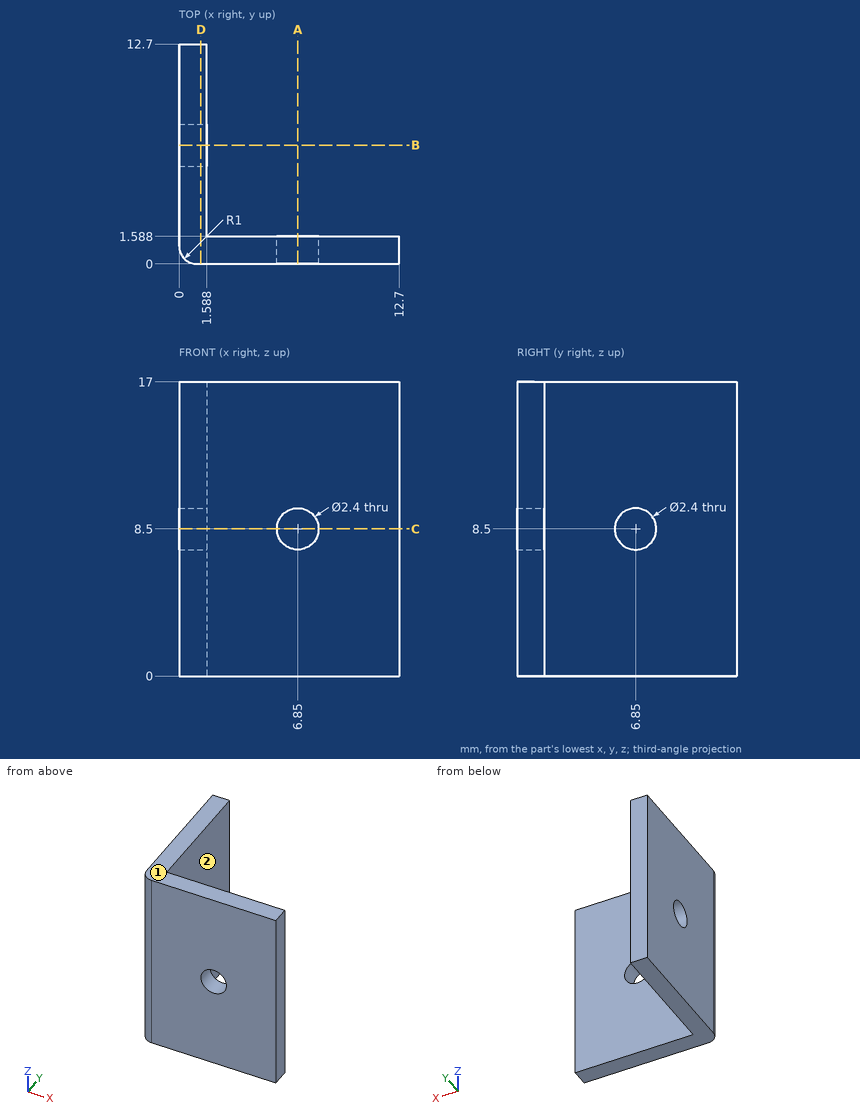
Can you work these out from the drawing? Everything is in mm from the part's minimum corner. A direction names the side the tool comes from. Round coordinates to 2 decimals unless told otherwise and drop trailing zeros. Loops run counter-clockwise (first coordinate to the right, second up) from the corner with the lowest first, then second, coordinate; pieces in that order, holes last. Notation, with made-up numbers: (18.25, 57) - (46.25, 57) arc R30 ccw to (46.25, 93) - close; hole circle Ø6 at (39.25, 61). An arc over 180 degrees is marked (long way). Write item = value, one per line. Start each with the question number.
(1) If we section it at A-A (x = 6.85): Please give me the cut outline in (y, z).
(2) For P1, Ø6, axis at x = 8.5, z = 11.5, coming from the +Y side; P2, Ø1, axis at y = 3.5, z = 9, coming from the +X side, each with a flat end and sliding along its axis, tell me the tip position at first contact or that it passes through.
(3) If we section it at D-D (x = 1.25): Please give me the cut outline in (y, z).
(4) If I drill on probe 1 along Z at (x, y) = (6.85, 1.1); probe 2 along Y at (x, z) = (1.1, 8.5), over which ranges is the centre line in solid material (lowest first)? Write a range as [from, to].
(5) For the marked faces 1 and 2, which set-ups out of +Z, -Z, +X, -X, +Y, -Y let a thin tool reach every point of the face, with its end or its side?
(6) If we section it at C-C (z = 8.5): Please give me the cut outline in (x, y).
Ans:
q1.outline = (0, 0) - (1.59, 0) - (1.59, 7.3) - (0, 7.3) - close; (0, 9.7) - (1.59, 9.7) - (1.59, 17) - (0, 17) - close
q2.P1 = 1.59
q2.P2 = 1.59
q3.outline = (0, 0) - (12.7, 0) - (12.7, 17) - (0, 17) - close; hole circle Ø2.4 at (6.85, 8.5)
q4.probe_1 = [0, 7.3], [9.7, 17]
q4.probe_2 = [0, 5.65], [8.05, 12.7]
q5.face_1 = +Z, +X, -X, +Y, -Y
q5.face_2 = +Z, -Z, +X, +Y
q6.outline = (0, 1) arc R1 ccw to (1, 0) - (5.65, 0) - (5.65, 1.59) - (1.59, 1.59) - (1.59, 5.65) - (0, 5.65) - close; (0, 8.05) - (1.59, 8.05) - (1.59, 12.7) - (0, 12.7) - close; (8.05, 0) - (12.7, 0) - (12.7, 1.59) - (8.05, 1.59) - close
